```python
from build123d import *

# Parameters (mm, degrees)
SKETCH_1_W      = 53
SKETCH_1_H      = 82
EXTRUDE_1_DEPTH = 9.5
EXTRUDE_2_DEPTH = 5.5


with BuildPart() as part:
    # Sketch 1 → Extrude 1 (new body)
    with BuildSketch(Plane.XY):
        with Locations((26.5, 41)):
            Rectangle(SKETCH_1_W, SKETCH_1_H)
    extrude(amount=EXTRUDE_1_DEPTH)

    # Sketch 1_3 → Extrude 2 (add)
    with BuildSketch(Plane.XY):
        with BuildLine():
            Line((0, 68.75), (-0.75, 68.75))
            ThreePointArc((-0.75, 68.75), (-1.5, 68), (-0.75, 67.25))
            Line((-0.75, 67.25), (0, 67.25))
            Line((0, 67.25), (0, 68.75))
        make_face()
        with BuildLine():
            Line((0, 13.25), (0, 14.75))
            Line((0, 14.75), (-0.75, 14.75))
            ThreePointArc((-0.75, 14.75), (-1.5, 14), (-0.75, 13.25))
            Line((-0.75, 13.25), (0, 13.25))
        make_face()
        with BuildLine():
            Line((8.75, 0), (7.25, 0))
            Line((7.25, 0), (7.25, -0.75))
            ThreePointArc((7.25, -0.75), (8, -1.5), (8.75, -0.75))
            Line((8.75, -0.75), (8.75, 0))
        make_face()
        with BuildLine():
            Line((27.25, -0.75), (27.25, 0))
            Line((27.25, 0), (25.75, 0))
            Line((25.75, 0), (25.75, -0.75))
            ThreePointArc((25.75, -0.75), (26.5, -1.5), (27.25, -0.75))
        make_face()
        with BuildLine():
            Line((45.75, -0.75), (45.75, 0))
            Line((45.75, 0), (44.25, 0))
            Line((44.25, 0), (44.25, -0.75))
            ThreePointArc((44.25, -0.75), (45, -1.5), (45.75, -0.75))
        make_face()
    extrude(amount=EXTRUDE_2_DEPTH)


solid = part.part
```
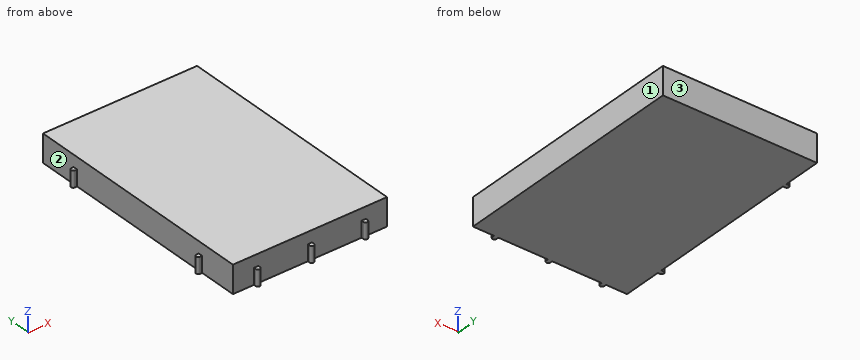
Model file for the job. Use its own axes, mm. Face numbers are marked on the shaded views. Coordinates: 2 decimals unless noted, no trailing zeros. Write each loop counter-clockwise with the first axis right and the second up, starting at its lowest first coordinate (ties: lowest second). Pieces come first, ordered by that corner, then holes. Notation, with made-up numbers: (27, -1.5) - (48, -1.5) arc R10 cw to (48, 5.5) - close; hole circle Ø2 at (-0.75, -19.75). An arc over 180 degrees is marked (long way). Use a Markdown table: item, result. Add a question column.
Item 1: Band-saw the part on B-B, the plane y = 70.5. Write the cut outline in (x, z).
Item 2: Drop flat-ended pins along their axis: pin 1 (1.5 mm diameter, centred on y = 10, z = 3.5, fed in from -X); pin 2 (0.8 mm diameter, centred on y = -0.5, z = 4, fed in from +X); pin 3 (0.6 mm diameter, centred on x = -0.5, z = 1.5, fed in from -Y). Give the stop position or say it passes through.
Item 3: Two-plate mould, pull along Y, no slides. Class the marked faces 1, 2 and 3: pulls with the +Y half, pulls with the -Y half, needs draft (parallel to the pull), parting line crosses it, or undercut.
Item 4: Band-saw the part on C-C, the plane x = 47. Write the cut outline in (y, z).
Item 5: Band-saw the part on A-A, the plane z = 3. Write the cut outline in (x, y), and give its area (3 significant figures).
Item 6: Drill centre lines: line 1 along X through (y, z) = (31, 5.25); line 2 along Y through (x, z) = (16, 3.25); line 3 along Y through (x, z) = (45.5, 3.5). Where is each one in solid material? Low to high.
A:
| question | item | result |
|---|---|---|
| 1 | outline | (0, 0) - (53, 0) - (53, 9.5) - (0, 9.5) - close |
| 2 | pin 1 | stops at x = 0 |
| 2 | pin 2 | stops at x = 45.75 |
| 2 | pin 3 | stops at y = 13.25 |
| 3 | face 1 | needs draft |
| 3 | face 2 | undercut |
| 3 | face 3 | pulls with the +Y half |
| 4 | outline | (0, 0) - (82, 0) - (82, 9.5) - (0, 9.5) - close |
| 5 | outline | (-0.75, 13.25) - (0, 13.25) - (0, 0) - (7.25, 0) - (7.25, -0.75) arc R0.75 ccw to (8.75, -0.75) - (8.75, 0) - (25.75, 0) - (25.75, -0.75) arc R0.75 ccw to (27.25, -0.75) - (27.25, 0) - (44.25, 0) - (44.25, -0.75) arc R0.75 ccw to (45.75, -0.75) - (45.75, 0) - (53, 0) - (53, 82) - (0, 82) - (0, 68.75) - (-0.75, 68.75) arc R0.75 ccw to (-0.75, 67.25) - (0, 67.25) - (0, 14.75) - (-0.75, 14.75) arc R0.75 ccw to start |
| 5 | area | 4,360 mm² |
| 6 | line 1 | x = 0 to 53 |
| 6 | line 2 | y = 0 to 82 |
| 6 | line 3 | y = -1.31 to 82 |
